Autodesk Inventor part; units mm, degrees
ref_plane "MP_XY" through (0, 0, 0) normal (0, 0, 1) x (1, 0, 0)
ref_plane "MP_YZ" through (0, 0, 0) normal (1, 0, 0) x (0, 1, 0)
ref_plane "MP_ZX" through (0, 0, 0) normal (0, 1, 0) x (0, 0, 1)
sketch "Sketch_11" plane through (0, 0, 0) normal (0, 0, 1) x (1, 0, 0)
  line L0 (-275, 698.5) -> (-275, 11.5)
  line L1 (-275, 11.5) -> (-274.0774, 11.5)
  arc A0 (-273.2113, 11) -> (-274.0774, 11.5) centre (-274.0774, 10.5) ccw
  line L2 (-273.2113, 11) -> (-264.2624, -4.5)
  arc A1 (-264.2624, -4.5) -> (-263.3964, -5) centre (-263.3964, -4) ccw
  line L3 (-263.3964, -5) -> (-256.5, -5)
  arc A2 (-256.5, -5) -> (-255.5, -4) centre (-256.5, -4) ccw
  line L4 (-255.5, -4) -> (-255.5, 0)
  arc A3 (-244.5, 0) -> (-255.5, 0) centre (-250, 0) ccw
  line L5 (-244.5, 0) -> (-244.5, -11)
  line L6 (-244.5, -11) -> (-243, -12.5)
  line L7 (-243, -12.5) -> (243, -12.5)
  line L8 (243, -12.5) -> (244.5, -11)
  line L9 (244.5, -11) -> (244.5, 0)
  arc A4 (255.5, 0) -> (244.5, 0) centre (250, 0) ccw
  line L10 (255.5, 0) -> (255.5, -4)
  arc A5 (255.5, -4) -> (256.5, -5) centre (256.5, -4) ccw
  line L11 (256.5, -5) -> (263.3964, -5)
  arc A6 (263.3964, -5) -> (264.2624, -4.5) centre (263.3964, -4) ccw
  line L12 (264.2624, -4.5) -> (273.2113, 11)
  arc A7 (274.0774, 11.5) -> (273.2113, 11) centre (274.0774, 10.5) ccw
  line L13 (274.0774, 11.5) -> (275, 11.5)
  line L14 (275, 11.5) -> (275, 698.5)
  line L15 (275, 698.5) -> (274.0774, 698.5)
  arc A8 (273.2113, 699) -> (274.0774, 698.5) centre (274.0774, 699.5) ccw
  line L16 (273.2113, 699) -> (264.2624, 714.5)
  arc A9 (264.2624, 714.5) -> (263.3964, 715) centre (263.3964, 714) ccw
  line L17 (263.3964, 715) -> (256.5, 715)
  arc A10 (256.5, 715) -> (255.5, 714) centre (256.5, 714) ccw
  line L18 (255.5, 714) -> (255.5, 710)
  arc A11 (244.5, 710) -> (255.5, 710) centre (250, 710) ccw
  line L19 (244.5, 710) -> (244.5, 721)
  line L20 (244.5, 721) -> (243, 722.5)
  line L21 (243, 722.5) -> (-243, 722.5)
  line L22 (-243, 722.5) -> (-244.5, 721)
  line L23 (-244.5, 721) -> (-244.5, 710)
  arc A12 (-255.5, 710) -> (-244.5, 710) centre (-250, 710) ccw
  line L24 (-255.5, 710) -> (-255.5, 714)
  arc A13 (-255.5, 714) -> (-256.5, 715) centre (-256.5, 714) ccw
  line L25 (-256.5, 715) -> (-263.3964, 715)
  arc A14 (-263.3964, 715) -> (-264.2624, 714.5) centre (-263.3964, 714) ccw
  line L26 (-264.2624, 714.5) -> (-273.2113, 699)
  arc A15 (-274.0774, 698.5) -> (-273.2113, 699) centre (-274.0774, 699.5) ccw
  line L27 (-274.0774, 698.5) -> (-275, 698.5)
  arc A16 (216.5296, 4.6222) -> (216.5296, -4.6222) centre (210, 0) ccw
  arc A17 (217.3457, -4.2) -> (216.5296, -4.6222) centre (217.3457, -5.2) ccw
  line L28 (217.3457, -4.2) -> (228, -4.2)
  arc A18 (228, -4.2) -> (229, -3.2) centre (228, -3.2) ccw
  line L29 (229, -3.2) -> (229, 3.2)
  arc A19 (229, 3.2) -> (228, 4.2) centre (228, 3.2) ccw
  line L30 (228, 4.2) -> (217.3457, 4.2)
  arc A20 (216.5296, 4.6222) -> (217.3457, 4.2) centre (217.3457, 5.2) ccw
  arc A21 (216.5296, 714.6222) -> (216.5296, 705.3778) centre (210, 710) ccw
  arc A22 (217.3457, 705.8) -> (216.5296, 705.3778) centre (217.3457, 704.8) ccw
  line L31 (217.3457, 705.8) -> (228, 705.8)
  arc A23 (228, 705.8) -> (229, 706.8) centre (228, 706.8) ccw
  line L32 (229, 706.8) -> (229, 713.2)
  arc A24 (229, 713.2) -> (228, 714.2) centre (228, 713.2) ccw
  line L33 (228, 714.2) -> (217.3457, 714.2)
  arc A25 (216.5296, 714.6222) -> (217.3457, 714.2) centre (217.3457, 715.2) ccw
  line L34 (-229, 3.2) -> (-229, -3.2)
  arc A26 (-229, -3.2) -> (-228, -4.2) centre (-228, -3.2) ccw
  line L35 (-228, -4.2) -> (-217.3457, -4.2)
  arc A27 (-216.5296, -4.6222) -> (-217.3457, -4.2) centre (-217.3457, -5.2) ccw
  arc A28 (-216.5296, -4.6222) -> (-216.5296, 4.6222) centre (-210, 0) ccw
  arc A29 (-217.3457, 4.2) -> (-216.5296, 4.6222) centre (-217.3457, 5.2) ccw
  line L36 (-217.3457, 4.2) -> (-228, 4.2)
  arc A30 (-228, 4.2) -> (-229, 3.2) centre (-228, 3.2) ccw
  arc A31 (-229, 706.8) -> (-228, 705.8) centre (-228, 706.8) ccw
  line L37 (-228, 705.8) -> (-217.3457, 705.8)
  arc A32 (-216.5296, 705.3778) -> (-217.3457, 705.8) centre (-217.3457, 704.8) ccw
  arc A33 (-216.5296, 705.3778) -> (-216.5296, 714.6222) centre (-210, 710) ccw
  arc A34 (-217.3457, 714.2) -> (-216.5296, 714.6222) centre (-217.3457, 715.2) ccw
  line L38 (-217.3457, 714.2) -> (-228, 714.2)
  arc A35 (-228, 714.2) -> (-229, 713.2) centre (-228, 713.2) ccw
  line L39 (-229, 713.2) -> (-229, 706.8)
extrude "Extrusion1" add sketch "Sketch_11" against normal blind 2.5
ref_plane "MP_XY" through (0, 0, 0) normal (0, 0, 1) x (1, 0, 0)
ref_plane "MP_YZ" through (0, 0, 0) normal (1, 0, 0) x (0, 1, 0)
ref_plane "MP_ZX" through (0, 0, 0) normal (0, 1, 0) x (0, 0, 1)
ref_plane "to_EB_XY" through (224.8, 0, -2.5) normal (0, 0, 1) x (1, 0, 0)
ref_plane "to_EB_YZ" through (224.8, 0, -2.5) normal (1, 0, 0) x (0, 1, 0)
ref_plane "to_EB_ZX" through (224.8, 0, -2.5) normal (0, 1, 0) x (0, 0, 1)
properties part number "1676X_02_00_P6_(1)"
Could you check a few things on this model? Use its own coordinates, in mm. Give positions to 0.01 mm unless a question says otherwise; leave off trailing zeros. Answer in a Markdown table with one row per item. Add a question column.
Item 1: I'm going to push flat-ended pins straight in: P1, Ø0.5, axis at x = -274.5, z = -2, coming from the -Y side; P2, Ø1.2, axis at x = -261, z = -1, coming from the -Y side; P3, Ø1.2, axis at y = 709.5, z = -0.5, coming from the -X side. Where does each tip first touch, or does it pass through?
Item 2: We'd pull the mould along Y, two halves only. Please class faces 1 (the cylindrical face through (-202, 0, -1)), 2 (the flat face through (-4, 360, 0)), 3 (the cylindrical face through (-202, 710, -1)): pulls with the +Y half, pulls with the -Y half, needs draft (parallel to the pull), parting line crosses it, or undercut.
Item 3: Please list where these lines run through material, in increasing order: probe 1 along Y at (x, z) = (210, -1.65); probe 2 along Y at (x, z) = (221, -0.4); probe 3 along X at (y, z) = (0, -0.9).
Result:
| question | item | result |
|---|---|---|
| 1 | P1 | y = 11.5 |
| 1 | P2 | y = -5 |
| 1 | P3 | x = -267.5 |
| 2 | face 1 | undercut |
| 2 | face 2 | needs draft |
| 2 | face 3 | undercut |
| 3 | probe 1 | -12.5 to -8, 8 to 702, 718 to 722.5 |
| 3 | probe 2 | -12.5 to -4.2, 4.2 to 705.8, 714.2 to 722.5 |
| 3 | probe 3 | -266.86 to -255.5, -244.5 to -229, -202 to 202, 229 to 244.5, 255.5 to 266.86 |
